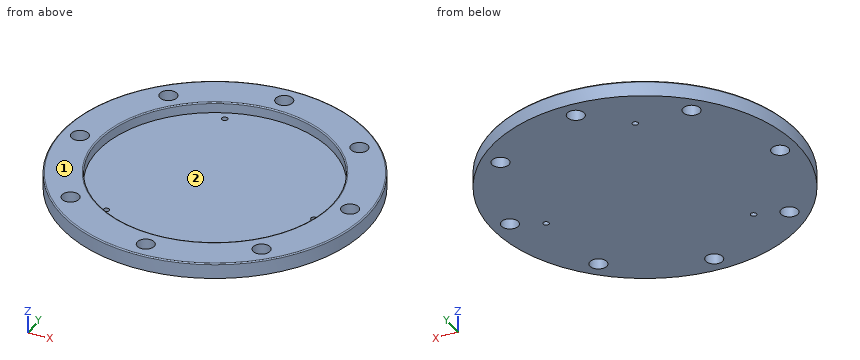
```python
from build123d import *

# Parameters (mm, degrees)
F2_R     = 76.454
F3_DEPTH = 6.35
F4_R     = 5.55625
F5_DEPTH = 10.161
F6_R     = 1.905
F7_DEPTH = 3.176


with BuildPart() as f1:
    # F0 (on Front) → F1 (revolve)
    with BuildSketch(Plane.XZ):
        with BuildLine():
            Line((0, 9.525), (0, 0))
            Line((0, 0), (100, 0))
            Line((100, 0), (100, 9.398))
            ThreePointArc((100, 9.398), (99.7768153673, 9.9368153673), (99.238, 10.16))
            Line((99.238, 10.16), (77.216, 10.16))
            ThreePointArc((77.216, 10.16), (76.6771846327, 9.9368153673), (76.454, 9.398))
            Line((76.454, 9.398), (76.454, 9.525))
            Line((76.454, 9.525), (0, 9.525))
        make_face()
    revolve(axis=Axis((0, 0, 85.8672061428), (0, 0, -1)))

    # F2 (on face) → F3 (cut)
    with BuildSketch(Plane.XY.offset(9.525)):
        Circle(F2_R)
    extrude(amount=-F3_DEPTH, mode=Mode.SUBTRACT)

    # F4 (on face) → F5 (cut, through all)
    with BuildSketch(Plane.XY.offset(10.16)):
        with Locations((0, 88.227)):
            Circle(F4_R)
        with Locations((-62.3859099837, 62.3859099837)):
            Circle(F4_R)
        with Locations((-88.227, 0)):
            Circle(F4_R)
        with Locations((-62.3859099837, -62.3859099837)):
            Circle(F4_R)
        with Locations((0, -88.227)):
            Circle(F4_R)
        with Locations((62.3859099837, -62.3859099837)):
            Circle(F4_R)
        with Locations((88.227, 0)):
            Circle(F4_R)
        with Locations((62.3859099837, 62.3859099837)):
            Circle(F4_R)
    extrude(amount=-F5_DEPTH, mode=Mode.SUBTRACT)

    # F6 (on face) → F7 (cut, through all)
    with BuildSketch(Plane.XY.offset(3.175)):
        with Locations((-26.7304377507, 64.5329853459)):
            Circle(F6_R)
        with Locations((-42.5219858163, -55.4157308193)):
            Circle(F6_R)
        with Locations((69.252423567, -9.1172545266)):
            Circle(F6_R)
    extrude(amount=-F7_DEPTH, mode=Mode.SUBTRACT)


solid = f1.part
```
Input: part model. Units: mm. Frame: model coordinates. Face numbers are marked on the shaded views. Give positions to 0.01 mm unless a question says otherwise; leave off trailing zeros. Loops run counter-clockwise (first coordinate to the right, second up) from the corner with the lowest first, then second, coordinate; pieces in that order, holes last. Notation, with made-up numbers: (-34, 78) -> (18, 78) arc R13 ccw to (18, 103) -> close; hole circle Ø11 at (49.5, -22.75). An arc over 180 degrees is marked (long way). Use a Markdown table: item, result.
Q1. Section query C-C, the plane z = 6.75. State how many separate pieces and enclosed holes the cut face has, plus the area to 3 significant figures.
Entries:
| item | result |
|---|---|
| separate pieces | 1 |
| enclosed holes | 9 |
| area | 12,300 mm² |
Q2. Section query A-A, the plane x = 0. Return the cut outline in (y, z) (3 decimals).
Entries:
| item | result |
|---|---|
| outline | (-100, 0) -> (-93.783, 0) -> (-93.783, 10.16) -> (-99.238, 10.16) arc R0.762 ccw to (-100, 9.398) -> close; (-82.671, 0) -> (82.671, 0) -> (82.671, 10.16) -> (77.216, 10.16) arc R0.762 ccw to (76.454, 9.398) -> (76.454, 3.175) -> (-76.454, 3.175) -> (-76.454, 9.398) arc R0.762 ccw to (-77.216, 10.16) -> (-82.671, 10.16) -> close; (93.783, 0) -> (100, 0) -> (100, 9.398) arc R0.762 ccw to (99.238, 10.16) -> (93.783, 10.16) -> close |
Q3. First-contact query: P1, Ø10, axis at x = 0, y = 88.227, coming from the +Z side; P2, Ø5, axis at x = 69.25, y = -9.12, coming from the +Z side (3 decimals); P3, Ø3, axis at y = 58, z = 3, coming from the +X side; P4, Ø3, axis at y = -72, z = 1.5, coming from the +X side. Flat tips, straight axial feed; report the tip coordinate or a pass-through.
Entries:
| item | result |
|---|---|
| P1 | passes through |
| P2 | stops at z = 3.175 |
| P3 | stops at x = 82.51 |
| P4 | stops at x = 70.92 |
Q4. Ray query, probe 1 along Y at (x, z) = (0, 6.25); probe 2 along X at (y, z) = (63.5, 3); probe 3 along Y at (x, z) = (-1.5, 1). Return the intervals inside material, ascending. Write a range as from..to.
Entries:
| item | result |
|---|---|
| probe 1 | y = -100..-93.78, -82.67..-76.45, 76.45..82.67, 93.78..100 |
| probe 2 | x = -77.25..-67.83, -56.94..-28.33, -25.13..56.94, 67.83..77.25 |
| probe 3 | y = -99.99..-93.58, -82.88..82.88, 93.58..99.99 |
Q5. Pull-direction query (X, two-part tool) for the marked faces 1 and 2; classes: pulls with the +X half, pulls with the -X half, needs draft (parallel to the pull), parting line crosses it, or undercut.
Entries:
| item | result |
|---|---|
| face 1 | needs draft |
| face 2 | undercut |
